The drawing under review shows one solid part. Ordinate dimensions are in mm from its lowest x, y, z. Round coordinates to 2 decimals unless told otherwise and drop trailing zeros. Order: outer loops, then holes, each group sorted by start corner. A loop starts at its lowest first (then second) coordinate and runs counter-clockwise, first axis right, second up. Notation, with made-up numbers: M 70,76 L 87,76 A22 ccw 87,86 Z; hole C 40.25,14 d3. An arc over 180 degrees is marked long. Answer as a JSON object with one key per item and string values. Group by question number.
1) To check wall thickness, follow line 1 (Y direction, x = 2.8, z = 215); line 2 (Z direction, x = 1.1, y = 29); line 3 (Z direction, x = 1.2, y = 122). State the ranges of each line that lie inside material, in increasing order.
2) Consider section B-B, the plane y = 30. Write out the cut boundary in (x, z), then the cut area to 4 significant figures.
3) Consider section A-A, the plane z = 215. Write out the cut boundary in (x, y), then the cut area to 3 significant figures.
4) Insertion check: pin 1 Ø10 at (y, z) = (79, 95.5) entering from -X; pin 2 Ø4.5 at (y, z) = (30, 215) entering from +X. Each pin has a flat end and moves straight along its axis. Give the tip position at first contact, or say it passes through.
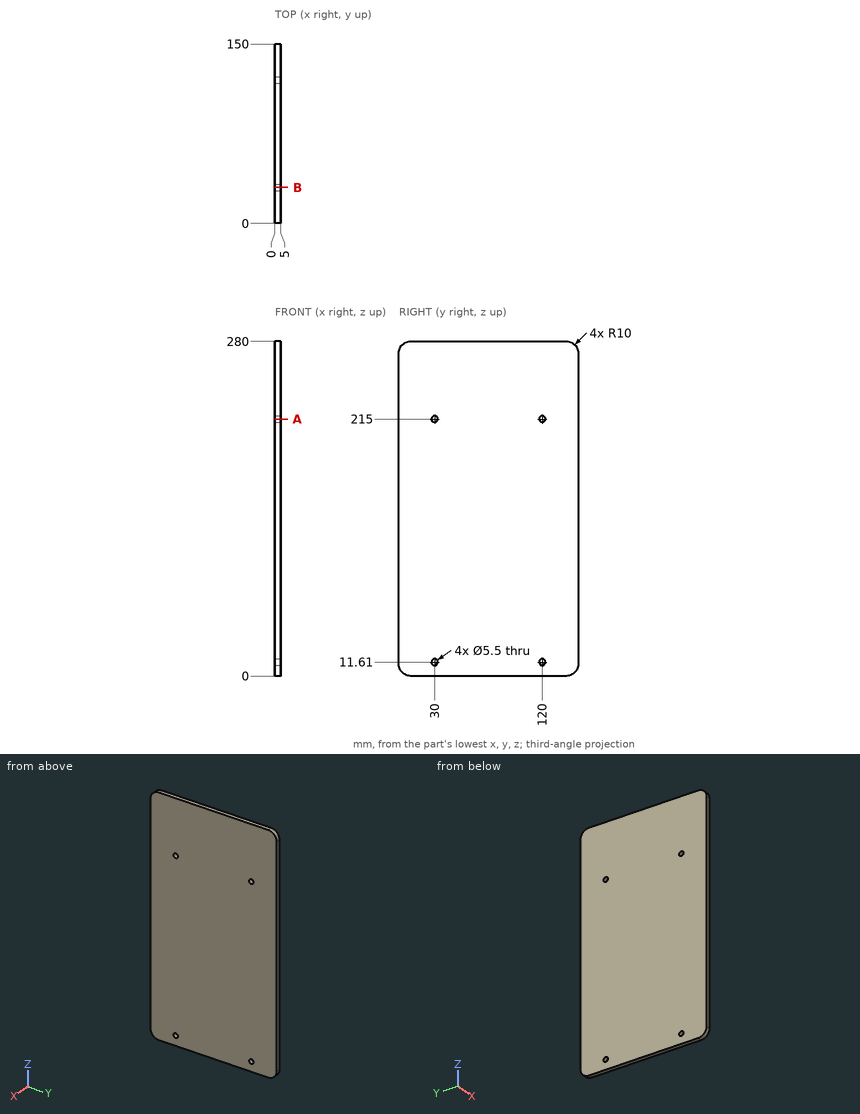
Results list:
{
 "1": {"line 1": "0 to 27.25, 32.75 to 117.25, 122.75 to 150", "line 2": "0 to 9.05, 14.17 to 212.44, 217.56 to 280", "line 3": "0 to 9.72, 13.5 to 213.11, 216.89 to 280"},
 "2": {"outline": "M 0,0 L 5,0 L 5,8.86 L 0,8.86 Z; M 0,14.36 L 5,14.36 L 5,212.25 L 0,212.25 Z; M 0,217.75 L 5,217.75 L 5,280 L 0,280 Z", "area": "1,345 mm^2"},
 "3": {"outline": "M 0,0 L 5,0 L 5,27.25 L 0,27.25 Z; M 0,32.75 L 5,32.75 L 5,117.25 L 0,117.25 Z; M 0,122.75 L 5,122.75 L 5,150 L 0,150 Z", "area": "695 mm^2"},
 "4": {"pin 1": "x = 0", "pin 2": "through"}
}
